Could you check a few things on this model? Use its own coordinates, in mm. Give positions to 0.01 mm unless a question says otherwise; leave off trailing zeros. Order: outer loops, then holes, each group sorted by start corner. A loop starts at its lowest first (then second) coordinate and runs counter-clockwise, first axis right, second up. Notation, with made-up numbers: (25.5, 30.25) -> (30.5, 30.25) arc R30 cw to (30.5, 64.25) -> close; hole circle Ø4 at (79, 35). An arc over 180 degrees is marked (long way). One line per item, written item: value.
Solid Edge part; units mm, degrees
sketch "Sketch1" plane through (0, 0, 0) normal (0, -1, 0) x (1, 0, 0)
  line L0 (-15, 41) -> (15, 41)
  line L1 (15, 41) -> (15, 35.1)
  line L2 (15, 35.1) -> (-15, 35.1)
  line L3 (-15, 35.1) -> (-15, 41)
  dimension "D1" = 15
revolve "RevolvedProtrusion1" add sketch "Sketch1" angle 360 about axis through (-60, 0, 0) along (1, 0, 0)
chamfer "Chamfer1" distance 1 angle 45 4 edges at (15, 0, -35.1) (15, 0, -41) (-15, 0, -41) (-15, 0, -35.1)
properties material "Polypropylene, general purpose"
1) We'd pull the mould along Z, two halves only. Please class faces 1 (the cylindrical face through (-0.2, -21.36, -27.85)), 2 (the flat face through (15, -36, -6)), 3 (the cylindrical face through (0, 40, -9)): +Z half, -Z half, draft (parallel to the pull), parting line (faces both ways), or undercut.
Answer below:
face 1: undercut
face 2: draft
face 3: parting line
2) For P1, Ø6, axis at x = -2, y = 32, coming from the -Z side; P2, Ø12, axis at y = -4, z = -29.5, coming from the -X side; P3, Ø6, axis at x = 0.5, y = -22.5, coming from the +Z side, each with a flat end and sliding along its axis, tell me the tip position at first contact or that it passes through.
Answer below:
P1: stops at z = -28.98
P2: stops at x = -14.67
P3: stops at z = 36.07
3) Suppose I cut it at A-A, the plane z = 0. Write out the boundary of the cut face in (x, y).
Answer below:
outline: (-15, -40) -> (-14, -41) -> (14, -41) -> (15, -40) -> (15, -36.1) -> (14, -35.1) -> (-14, -35.1) -> (-15, -36.1) -> close; (-15, 36.1) -> (-14, 35.1) -> (14, 35.1) -> (15, 36.1) -> (15, 40) -> (14, 41) -> (-14, 41) -> (-15, 40) -> close
4) If I drill on line 1 along Z through (x, y) = (-5, 0); line 2 along Z through (x, y) = (2.75, -3), over which ranges is the centre line in solid material (lowest first)?
Answer below:
line 1: z = -41 to -35.1, 35.1 to 41
line 2: z = -40.89 to -34.97, 34.97 to 40.89
5) Suppose I cut it at C-C, the plane x = 5. Write out the boundary of the cut face in (y, z), then the cut area to 3 significant figures.
Answer below:
outline: circle Ø82 at (0, 0); hole circle Ø70.2 at (0, 0)
area: 1,410 mm2
